Can you work these out from the model? Positions are in its coordinate system, mm. A direction names the side the tool comes from. Give positions to 0.01 mm unless a question says otherwise; leave off trailing zeros. Write each loop counter-clockwise with the first axis right and the second up, starting at its lowest first coordinate (ties: lowest second). Pieces come first, ordered by that corner, then holes.
1. On a 3-axis mill with a long thin cutter (end or side, diameter ignored), from which of +Z, -Z, +X, -X, +Y, -Y can I reach the whole of each face in a straight line? I mean faces 3 (the flat face through (45, 17, -34)), 4 (the cylindrical face through (45.71, 19.1, -63.76)), 5 (the cylindrical face through (94.583, 6.591, -9.759)), 6 (the flat face through (115.945, 16.83, -83.027)). Say none if no direction works.
2. Suppose I cut it at B-B (y = 6.5). Please give me the cut outline in (x, z).
3. Suppose I cut it at C-C (x = 140). Give the number of separate pieces and of enclosed holes in the cut face, and give its area (3 significant figures).
4. If I drill on probe 1 along X at (y, z) = (5.5, -9); probe 2 along Z at (x, y) = (178, 7.25); probe 3 along X at (y, z) = (15.75, -98), over which ranges is the centre line in solid material (lowest first)?
5. Suppose I cut it at A-A (z = -53.5). Please give me the cut outline in (x, y), and give its area (3 significant figures).
6. Thinking about a two-plate mould opening in Z: for faces 1 (the flat face through (97, 10, 0)), 2 (the flat face through (15, 13, -95)), which applies, pulls with the +Z half, pulls with the -Z half, needs draft (parallel to the pull), parting line crosses it, or undercut?
7. I'm going to push flat-ended pins straight in: pin 1 (13.5 mm diameter, centred on x = 82.5, z = -58.5, fed in from -Y); pin 2 (6.5 mm diameter, centred on x = 21, z = -10.5, fed in from +Y); pin 3 (7.5 mm diameter, centred on x = 98, z = -9, fed in from +Y). Where does each tip first touch, or does it pass through?
```python
from build123d import *

# Parameters (mm, degrees)
SKETCH1_W           = 197
SKETCH1_H           = 107
BOSS_EXTRUDE1_DEPTH = 30
CUT_EXTRUDE1_DEPTH  = 227.181343174
SKETCH4_W           = 182
SKETCH4_H           = 45
CUT_EXTRUDE2_DEPTH  = 10
CUT_EXTRUDE3_DEPTH  = 164
SKETCH19_W          = 141.2
SKETCH19_H          = 21.2
CUT_EXTRUDE15_DEPTH = 1.4
SKETCH6_W           = 141.2
SKETCH6_H           = 21.2
CUT_EXTRUDE4_DEPTH  = 1.4
CUT_EXTRUDE5_REACH  = 228.181
SKETCH9_R           = 8
CUT_EXTRUDE6_DEPTH  = 171
SKETCH10_R          = 10
CUT_EXTRUDE7_DEPTH  = 1.5
SKETCH11_R          = 4.8
CUT_EXTRUDE8_DEPTH  = 12.5
SKETCH12_R          = 6.35
CUT_EXTRUDE9_DEPTH  = 17
CUT_EXTRUDE13_REACH = 225.36
SKETCH17_R          = 3.5
CUT_EXTRUDE14_DEPTH = 227.181343174
CUT_EXTRUDE16_REACH = 228.847


with BuildPart() as part:
    # Sketch1 → Boss-Extrude1 (new body)
    with BuildSketch(Plane(origin=(0, 0, 0), x_dir=(1, 0, 0), z_dir=(0, 1, 0))):
        with Locations((98.5, 53.5)):
            Rectangle(SKETCH1_W, SKETCH1_H)
    extrude(amount=BOSS_EXTRUDE1_DEPTH)

    # Sketch3 → Cut-Extrude1 (cut, through all)
    with BuildSketch(Plane(origin=(0, 30, 0), x_dir=(1, 0, 0), z_dir=(0, 1, 0))):
        Polygon((0, 0), (6.1, 0), (0, 6.1), align=None)
        Polygon((0, 107), (6.1, 107), (0, 100.9), align=None)
        Polygon((197, 100.9), (197, 107), (190.9, 107), align=None)
        Polygon((197, 6.1), (197, 0), (190.9, 0), align=None)
    extrude(amount=-CUT_EXTRUDE1_DEPTH, mode=Mode.SUBTRACT)

    # Sketch4 → Cut-Extrude2 (cut)
    with BuildSketch(Plane(origin=(0, 0, 0), x_dir=(1, 0, 0), z_dir=(0, 1, 0))):
        with Locations((98.5, 53.5)):
            Rectangle(SKETCH4_W, SKETCH4_H)
    extrude(amount=CUT_EXTRUDE2_DEPTH, mode=Mode.SUBTRACT)

    # Sketch5 → Cut-Extrude3 (cut)
    with BuildSketch(Plane(origin=(197, 0, 0), x_dir=(0, 0, -1), z_dir=(1, 0, 0))):
        Polygon((58.5, 30), (107, 17.907591862), (107, 30), align=None)
        Polygon((0, 17.907591862), (0, 30), (48.5, 30), align=None)
    extrude(amount=-CUT_EXTRUDE3_DEPTH, mode=Mode.SUBTRACT)

    # Sketch19 → Cut-Extrude15 (cut)
    with BuildSketch(Plane(origin=(0, 16.859528495, 4.203552569), x_dir=(1, 0, 0), z_dir=(0, 0.9702957262759979, 0.2419218955996617))):
        with BuildLine():
            Line((45, 24.332238569), (185, 24.332238569))
            ThreePointArc((185, 24.332238569), (187.121320344, 25.210918225), (188, 27.332238569))
            Line((188, 27.332238569), (188, 47.332238569))
            ThreePointArc((188, 47.332238569), (187.121320344, 49.453558912), (185, 50.332238569))
            Line((185, 50.332238569), (45, 50.332238569))
            ThreePointArc((45, 50.332238569), (42.878679656, 49.453558912), (42, 47.332238569))
            Line((42, 47.332238569), (42, 27.332238569))
            ThreePointArc((42, 27.332238569), (42.878679656, 25.210918225), (45, 24.332238569))
        make_face()
        with Locations((115, 37.332238569)):
            Rectangle(SKETCH19_W, SKETCH19_H, mode=Mode.SUBTRACT)
    extrude(amount=-CUT_EXTRUDE15_DEPTH, mode=Mode.SUBTRACT)

    # Sketch6 → Cut-Extrude4 (cut)
    with BuildSketch(Plane(origin=(0, 41.976257104, -10.465856351), x_dir=(1, 0, 0), z_dir=(0, 0.9702957262759981, -0.24192189559966115))):
        with BuildLine():
            Line((45, 79.489404143), (185, 79.489404143))
            ThreePointArc((185, 79.489404143), (187.121320344, 78.610724486), (188, 76.489404143))
            Line((188, 76.489404143), (188, 56.489404143))
            ThreePointArc((188, 56.489404143), (187.121320344, 54.368083799), (185, 53.489404143))
            Line((185, 53.489404143), (45, 53.489404143))
            ThreePointArc((45, 53.489404143), (42.878679656, 54.368083799), (42, 56.489404143))
            Line((42, 56.489404143), (42, 76.489404143))
            ThreePointArc((42, 76.489404143), (42.878679656, 78.610724486), (45, 79.489404143))
        make_face()
        with Locations((115, 66.489404143)):
            Rectangle(SKETCH6_W, SKETCH6_H, mode=Mode.SUBTRACT)
    extrude(amount=-CUT_EXTRUDE4_DEPTH, mode=Mode.SUBTRACT)

    # Cut-Extrude5: up to this face of the body (flat: up to its plane)
    cut_extrude5_end = Plane(part.part.faces().sort_by_distance((33, 25.969197287, -90.833333333))[0])
    # Sketch7 → Cut-Extrude5 (cut, up to the picked face)
    with BuildSketch(Plane(origin=(0, 0, 0), x_dir=(0, 0, -1), z_dir=(1, 0, 0)), mode=Mode.PRIVATE) as cut_extrude5_sk1:
        Polygon((107, 30), (107, 25), (82.505102572, 30), align=None)
    cut_extrude5_tool1 = split(extrude(cut_extrude5_sk1.sketch, amount=CUT_EXTRUDE5_REACH, mode=Mode.PRIVATE), bisect_by=cut_extrude5_end, keep=Keep.BOTH, mode=Mode.PRIVATE)
    # Sketch7 → Cut-Extrude5 (cut, up to the picked face)
    with BuildSketch(Plane(origin=(0, 0, 0), x_dir=(0, 0, -1), z_dir=(1, 0, 0)), mode=Mode.PRIVATE) as cut_extrude5_sk2:
        Polygon((0, 25), (0, 30), (24.494897428, 30), align=None)
    cut_extrude5_tool2 = split(extrude(cut_extrude5_sk2.sketch, amount=CUT_EXTRUDE5_REACH, mode=Mode.PRIVATE), bisect_by=cut_extrude5_end, keep=Keep.BOTH, mode=Mode.PRIVATE)
    add(cut_extrude5_tool1.solids().sort_by(Axis((0, 28.333333, -98.835034), (1, 0, 0)))[0], mode=Mode.SUBTRACT)
    add(cut_extrude5_tool2.solids().sort_by(Axis((0, 28.333333, -8.164966), (1, 0, 0)))[0], mode=Mode.SUBTRACT)

    # Sketch9 → Cut-Extrude6 (cut)
    with BuildSketch(Plane(origin=(0, 30, 0), x_dir=(1, 0, 0), z_dir=(0, 1, 0))):
        with Locations(Location((16, 53.5, 0), (0, 0, 270))):
            Circle(SKETCH9_R)
    extrude(amount=-CUT_EXTRUDE6_DEPTH, mode=Mode.SUBTRACT)

    # Sketch10 → Cut-Extrude7 (cut)
    with BuildSketch(Plane(origin=(0, 30, 0), x_dir=(1, 0, 0), z_dir=(0, 1, 0))):
        with Locations(Location((16, 53.5, 0), (0, 0, 270))):
            Circle(SKETCH10_R)
    extrude(amount=-CUT_EXTRUDE7_DEPTH, mode=Mode.SUBTRACT)

    # Sketch11 → Cut-Extrude8 (cut)
    with BuildSketch(Plane(origin=(0, 30, 0), x_dir=(1, 0, 0), z_dir=(0, 1, 0))):
        with Locations(Location((16, 72.905102572, 0), (0, 0, 270))):
            Circle(SKETCH11_R)
        with Locations(Location((16, 34.094897428, 0), (0, 0, 270))):
            Circle(SKETCH11_R)
    extrude(amount=-CUT_EXTRUDE8_DEPTH, mode=Mode.SUBTRACT)

    # Sketch12 → Cut-Extrude9 (cut)
    with BuildSketch(Plane(origin=(0, 30, 0), x_dir=(1, 0, 0), z_dir=(0, 1, 0))):
        with Locations(Location((18, 98, 0), (0, 0, 270))):
            Circle(SKETCH12_R)
        with Locations(Location((98, 9, 0), (0, 0, 270))):
            Circle(SKETCH12_R)
        with Locations(Location((178, 9, 0), (0, 0, 270))):
            Circle(SKETCH12_R)
        with Locations(Location((18, 9, 0), (0, 0, 270))):
            Circle(SKETCH12_R)
        with Locations(Location((98, 98, 0), (0, 0, 270))):
            Circle(SKETCH12_R)
        with Locations(Location((178, 98, 0), (0, 0, 270))):
            Circle(SKETCH12_R)
    extrude(amount=-CUT_EXTRUDE9_DEPTH, mode=Mode.SUBTRACT)

    # Cut-Extrude13: up to this plane
    cut_extrude13_end = Plane(origin=(0, 10, 0), z_dir=(0, -1, 0))
    # Sketch16 → Cut-Extrude13 (cut, up to the surface)
    with BuildSketch(Plane(origin=(0, 41.976257104, -10.465856351), x_dir=(1, 0, 0), z_dir=(0, 0.9702957262759981, -0.24192189559966115)), mode=Mode.PRIVATE) as cut_extrude13_sk1:
        with BuildLine():
            Line((47.5, 56.489404143), (182.5, 56.489404143))
            ThreePointArc((182.5, 56.489404143), (184.267766953, 57.22163719), (185, 58.989404143))
            Line((185, 58.989404143), (185, 73.989404143))
            ThreePointArc((185, 73.989404143), (184.267766953, 75.757171096), (182.5, 76.489404143))
            Line((182.5, 76.489404143), (47.5, 76.489404143))
            ThreePointArc((47.5, 76.489404143), (45.732233047, 75.757171096), (45, 73.989404143))
            Line((45, 73.989404143), (45, 58.989404143))
            ThreePointArc((45, 58.989404143), (45.732233047, 57.22163719), (47.5, 56.489404143))
        make_face()
    cut_extrude13_tool1 = split(extrude(cut_extrude13_sk1.sketch, amount=-CUT_EXTRUDE13_REACH, mode=Mode.PRIVATE), bisect_by=cut_extrude13_end, keep=Keep.BOTH, mode=Mode.PRIVATE)
    add(cut_extrude13_tool1.solids().sort_by_distance((115, 25.891014, -74.980241))[0], mode=Mode.SUBTRACT)

    # Sketch17 → Cut-Extrude14 (cut, through all)
    with BuildSketch(Plane(origin=(0, 30, 0), x_dir=(1, 0, 0), z_dir=(0, 1, 0))):
        with Locations(Location((18, 9, 0), (0, 0, 270))):
            Circle(SKETCH17_R)
        with Locations(Location((18, 98, 0), (0, 0, 270))):
            Circle(SKETCH17_R)
        with Locations(Location((98, 98, 0), (0, 0, 270))):
            Circle(SKETCH17_R)
        with Locations(Location((178, 98, 0), (0, 0, 270))):
            Circle(SKETCH17_R)
        with Locations(Location((178, 9, 0), (0, 0, 270))):
            Circle(SKETCH17_R)
        with Locations(Location((98, 9, 0), (0, 0, 270))):
            Circle(SKETCH17_R)
    extrude(amount=-CUT_EXTRUDE14_DEPTH, mode=Mode.SUBTRACT)

    # Cut-Extrude16: up to this plane
    cut_extrude16_end = Plane(origin=(0, 10, 0), z_dir=(0, -1, 0))
    # Sketch20 → Cut-Extrude16 (cut, up to the surface)
    with BuildSketch(Plane(origin=(0, 16.859528495, 4.203552569), x_dir=(1, 0, 0), z_dir=(0, 0.9702957262759979, 0.2419218955996617)), mode=Mode.PRIVATE) as cut_extrude16_sk1:
        with BuildLine():
            Line((47.5, 27.332238569), (182.5, 27.332238569))
            ThreePointArc((182.5, 27.332238569), (184.267766953, 28.064471616), (185, 29.832238569))
            Line((185, 29.832238569), (185, 44.832238569))
            ThreePointArc((185, 44.832238569), (184.267766953, 46.600005522), (182.5, 47.332238569))
            Line((182.5, 47.332238569), (47.5, 47.332238569))
            ThreePointArc((47.5, 47.332238569), (45.732233047, 46.600005522), (45, 44.832238569))
            Line((45, 44.832238569), (45, 29.832238569))
            ThreePointArc((45, 29.832238569), (45.732233047, 28.064471616), (47.5, 27.332238569))
        make_face()
    cut_extrude16_tool1 = split(extrude(cut_extrude16_sk1.sketch, amount=-CUT_EXTRUDE16_REACH, mode=Mode.PRIVATE), bisect_by=cut_extrude16_end, keep=Keep.BOTH, mode=Mode.PRIVATE)
    add(cut_extrude16_tool1.solids().sort_by_distance((115, 25.891014, -32.019759))[0], mode=Mode.SUBTRACT)


solid = part.part
```
Checks:
1. face 3: none
1. face 4: -Y
1. face 5: +Y, -Y
1. face 6: +Y
2. outline: (0, -100.9) - (6.1, -107) - (190.9, -107) - (197, -100.9) - (197, -6.1) - (190.9, 0) - (6.1, 0) - (0, -6.1) - close; hole (7.5, -76) - (189.5, -76) - (189.5, -31) - (7.5, -31) - close; hole circle Ø7 at (18, -98); hole circle Ø7 at (18, -9); hole circle Ø7 at (98, -98); hole circle Ø7 at (98, -9); hole circle Ø7 at (178, -98); hole circle Ø7 at (178, -9)
3. separate pieces: 3
3. enclosed holes: 0
3. area: 1,500 mm2
4. probe 1: x = 0 to 14.5, 21.5 to 94.5, 101.5 to 174.5, 181.5 to 197
4. probe 2: z = -107 to -101.5, -94.5 to -76, -31 to -12.5, -5.5 to 0
4. probe 3: x = 0 to 11.65, 24.35 to 91.65, 104.35 to 171.65, 184.35 to 197
5. outline: (0, 0) - (7.5, 0) - (7.5, 10) - (8, 10) - (8, 28.5) - (6, 28.5) - (6, 30) - (0, 30) - close; (24, 10) - (189.5, 10) - (189.5, 0) - (197, 0) - (197, 30) - (26, 30) - (26, 28.5) - (24, 28.5) - close
5. area: 3,760 mm2
6. face 1: pulls with the +Z half
6. face 2: undercut
7. pin 1: stops at y = 10
7. pin 2: stops at y = 27.71
7. pin 3: stops at y = 13
